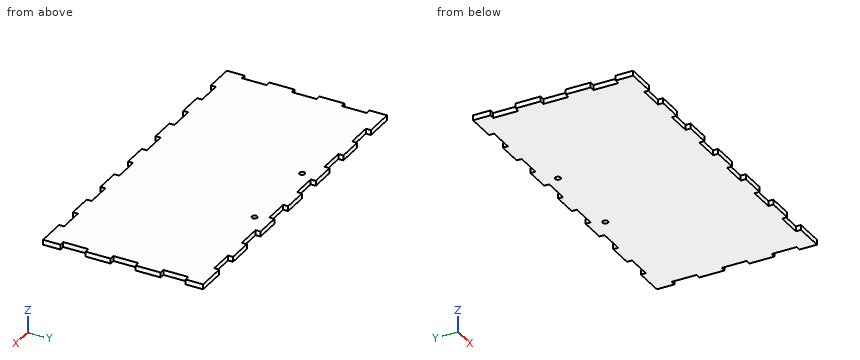
Autodesk Inventor part; units mm, degrees
ref_plane "Work Plane1" through (0, 0, 0) normal (0, 0, 1) x (1, 0, 0)
ref_plane "YZ Plane" through (0, 0, 0) normal (1, 0, 0) x (0, 1, 0)
ref_plane "XZ Plane" through (0, 0, 0) normal (0, 1, 0) x (-1, 0, 0)
ref_plane "Work Plane1" through (0, 0, 0) normal (0, 0, 1) x (1, 0, 0)
sketch "Sketch1" plane through (0, 0, 0) normal (0, 0, 1) x (1, 0, 0)
  line L0 (0, -5) -> (43, -5)
  line L1 (0, -25) -> (0, -5)
  line L2 (0, -25) -> (3, -25)
  line L3 (3, -25) -> (43, -25)
  line L4 (43, -5) -> (43, -25)
  line L5 (127, -5) -> (170, -5)
  line L6 (127, -5) -> (127, -25)
  line L7 (167, -25) -> (127, -25)
  line L8 (170, -25) -> (167, -25)
  line L9 (170, -25) -> (170, -5)
  ellipse E0 centre (272.0385, -161.4535) end of major axis (262.0385, -161.4535) minor radius 9.7437
  line L10 (264.0385, -174.9547) -> (285, -186.7467)
  line L11 (285, -186.7467) -> (285, -136.1602)
  line L12 (285, -136.1602) -> (264.0385, -147.9522)
  ellipse E1 centre (272.0385, -161.4535) end of major axis (256.0385, -161.4535) minor radius 15.5899 (264.0385, -147.9522) -> (264.0385, -174.9547) ccw
  ellipse E2 centre (-102.0385, -161.4535) end of major axis (-92.0385, -161.4535) minor radius 9.7437
  line L13 (-94.0385, -174.9547) -> (-115, -186.7467)
  ellipse E3 centre (-102.0385, -161.4535) end of major axis (-86.0385, -161.4535) minor radius 15.5899 (-94.0385, -174.9547) -> (-94.0385, -147.9522) ccw
  line L14 (-115, -136.1602) -> (-94.0385, -147.9522)
  line L15 (-115, -186.7467) -> (-115, -136.1602)
  line L16 (-115, -136.1602) -> (-115, -5) construction
  line L17 (-115, -5) -> (285, -5) construction
  line L18 (285, -5) -> (285, -186.7467) construction
  line L19 (285, -186.7467) -> (-115, -186.7467) construction
  line L20 (-115, -186.7467) -> (-115, -136.1602) construction
  line L21 (285, -5) -> (-115, -5)
  line L22 (-115, -5) -> (-115, -186.7467)
  line L23 (-115, -186.7467) -> (285, -186.7467)
  line L24 (285, -186.7467) -> (285, -5)
  circle A0 centre (147, -15) radius 3.25
  circle A1 centre (23, -15) radius 3.25
  circle A2 centre (23, -15) radius 2.4585
  circle A3 centre (147, -15) radius 2.4585
  line L25 (-115, -5) -> (285, -5)
  line L26 (285, -5) -> (285, 5)
  line L27 (285, 5) -> (-115, 5)
  line L28 (-115, 5) -> (-115, -5)
  point P0 (0, 0)
  point P1 (170, -15)
  point P2 (147, -25)
  point P3 (23, -25)
  point P4 (43, -15)
  dimension "d0" = 6.5
  dimension "d2" = 10
extrude "Plate1" add sketch "Sketch1" along normal blind 6 contours L21 L28 L27 L26 L5 L0 | L0 L4 L3 L2 L1 | L1 L2 L3 L4 L21 L6 L7 L8 L9 L24 L12 E1 L10 L23 L13 E3 L14 L22 | L5 L9 L8 L7 L6 | L14 E3 L13 L15 | L10 E1 L12 L11 | E0 | E2 | A0 | A1 | A2 | A3
sketch "Sketch2" plane through (0, 0, 6) normal (0, 0, 1) x (1, 0, 0)
  line L0 (-115, -186.7467) -> (-115, 5)
  line L1 (285, -186.7467) -> (-115, -186.7467)
  line L2 (285, 5) -> (285, -186.7467)
  line L3 (-115, 5) -> (285, 5)
  line L4 (285, -186.7467) -> (285, 5)
  line L5 (285, -75.8734) -> (279, -75.8734)
  line L6 (279, -75.8734) -> (279, -105.8734)
  line L7 (279, -105.8734) -> (285, -105.8734)
  line L8 (285, -105.8734) -> (285, -75.8734)
  line L9 (285, -45.8734) -> (279, -45.8734)
  line L10 (279, -45.8734) -> (279, -15.8734)
  line L11 (279, -15.8734) -> (285, -15.8734)
  line L12 (285, -15.8734) -> (285, -45.8734)
  line L13 (285, -135.8734) -> (279, -135.8734)
  line L14 (279, -135.8734) -> (279, -165.8734)
  line L15 (279, -165.8734) -> (285, -165.8734)
  line L16 (285, -165.8734) -> (285, -135.8734)
  line L17 (285, 5) -> (-115, 5) construction
  line L18 (85, 5) -> (85, -186.7467) construction
  line L19 (-115, -75.8734) -> (-109, -75.8734)
  line L20 (-109, -75.8734) -> (-109, -105.8734)
  line L21 (-109, -105.8734) -> (-115, -105.8734)
  line L22 (-115, -105.8734) -> (-115, -75.8734)
  line L23 (-115, -45.8734) -> (-109, -45.8734)
  line L24 (-109, -45.8734) -> (-109, -15.8734)
  line L25 (-109, -15.8734) -> (-115, -15.8734)
  line L26 (-115, -15.8734) -> (-115, -45.8734)
  line L27 (-115, -135.8734) -> (-109, -135.8734)
  line L28 (-109, -135.8734) -> (-109, -165.8734)
  line L29 (-109, -165.8734) -> (-115, -165.8734)
  line L30 (-115, -165.8734) -> (-115, -135.8734)
  line L31 (-115, -186.7467) -> (285, -186.7467)
  line L32 (250, -186.7467) -> (220, -186.7467)
  line L33 (220, -186.7467) -> (220, -180.7467)
  line L34 (220, -180.7467) -> (250, -180.7467)
  line L35 (250, -180.7467) -> (250, -186.7467)
  line L36 (190, -186.7467) -> (160, -186.7467)
  line L37 (160, -186.7467) -> (160, -180.7467)
  line L38 (160, -180.7467) -> (190, -180.7467)
  line L39 (190, -180.7467) -> (190, -186.7467)
  line L40 (130, -186.7467) -> (100, -186.7467)
  line L41 (100, -186.7467) -> (100, -180.7467)
  line L42 (100, -180.7467) -> (130, -180.7467)
  line L43 (130, -180.7467) -> (130, -186.7467)
  line L44 (285, -90.8734) -> (-115, -90.8734) construction
  line L45 (250, 5) -> (220, 5)
  line L46 (220, 5) -> (220, -1)
  line L47 (220, -1) -> (250, -1)
  line L48 (250, -1) -> (250, 5)
  line L49 (190, 5) -> (160, 5)
  line L50 (160, 5) -> (160, -1)
  line L51 (160, -1) -> (190, -1)
  line L52 (190, -1) -> (190, 5)
  line L53 (130, 5) -> (100, 5)
  line L54 (100, 5) -> (100, -1)
  line L55 (100, -1) -> (130, -1)
  line L56 (130, -1) -> (130, 5)
  circle A0 centre (23, -15) radius 3.25
  line L57 (-80, -186.7467) -> (-50, -186.7467)
  line L58 (-50, -186.7467) -> (-50, -180.7467)
  line L59 (-50, -180.7467) -> (-80, -180.7467)
  line L60 (-80, -180.7467) -> (-80, -186.7467)
  line L61 (-20, -186.7467) -> (10, -186.7467)
  line L62 (10, -186.7467) -> (10, -180.7467)
  line L63 (10, -180.7467) -> (-20, -180.7467)
  line L64 (-20, -180.7467) -> (-20, -186.7467)
  line L65 (40, -186.7467) -> (70, -186.7467)
  line L66 (70, -186.7467) -> (70, -180.7467)
  line L67 (70, -180.7467) -> (40, -180.7467)
  line L68 (40, -180.7467) -> (40, -186.7467)
  line L69 (70, 5) -> (70, -1)
  line L70 (40, 5) -> (70, 5)
  line L71 (40, -1) -> (40, 5)
  line L72 (10, 5) -> (10, -1)
  line L73 (-20, 5) -> (10, 5)
  line L74 (10, -1) -> (-20, -1)
  line L75 (-20, -1) -> (-20, 5)
  line L76 (70, -1) -> (40, -1)
  line L77 (-50, 5) -> (-50, -1)
  line L78 (-80, 5) -> (-50, 5)
  line L79 (-80, -1) -> (-80, 5)
  line L80 (-50, -1) -> (-80, -1)
  point P0 (0, 0)
  point P1 (115, -180.7467)
  point P2 (115, -1)
  point P3 (55, -180.7467)
  point P4 (55, -1)
  dimension "d3" = 6
  dimension "d4" = 30
  dimension "d5" = 30
  dimension "d6" = 30
  dimension "d7" = 30
  dimension "d8" = 30
  dimension "d10" = 15
extrude "Cut1" cut sketch "Sketch2" against normal blind 6 contours L0 L27 L28 L29 | L60 L59 L58 L1 | L0 L19 L20 L21 | L64 L63 L62 L1 | L0 L25 L24 L23 | L68 L67 L66 L1 | L41 L42 L43 L1 | L3 L77 L80 L79 | L37 L38 L39 L1 | L3 L72 L74 L75 | L33 L34 L35 L1 | L3 L69 L76 L71 | L3 L56 L55 L54 | L15 L14 L13 L2 | L3 L52 L51 L50 | L7 L6 L5 L2 | L3 L48 L47 L46 | L9 L10 L11 L2
sketch "Sketch3" plane through (0, 0, 0) normal (0, 0, -1) x (-1, 0, 0)
  circle A0 centre (-147, -15) radius 3.25
  circle A1 centre (-23, -15) radius 3.25
  circle A2 centre (-136.75, -15) radius 3.25
  circle A3 centre (-33.25, -15) radius 3.25
  line L0 (115, -5) -> (-285, -5) construction
  line L1 (-136.75, -15) -> (-33.25, -15) construction
  point P0 (0, 0)
  point P1 (-23, -15)
  point P2 (-85, -15)
  point P3 (-85, -5)
  dimension "d13" = 103.5
extrude "Cut2" cut sketch "Sketch3" against normal blind 6 contours A2 | A3
equation "\"d5\" = d4"
equation "\"d6\" = d5"
equation "\"d7\" = d4"
equation "\"d8\" = d7"
equation "\"d11\" = Thickness"
equation "\"d14\" = Thickness"
equation "\"d1\" = Thickness"
equation "\"BendRadius\" = Thickness"
equation "\"BendReliefWidth\" = Thickness"
equation "\"BendReliefDepth\" = 0.5 * Thickness"
equation "\"CornerReliefSize\" = 4 * Thickness"
equation "\"MinimumRemnant\" = 2 * Thickness"
equation "\"TransitionRadius\" = BendRadius"
equation "\"JacobiRadiusSize\" = BendRadius"
equation "\"GapSize\" = Thickness"
properties part number "elektronica behuizing" material "Wood (Birch)"
Design review of the part built by this model. Coordinates are the model's own, in mm. Coordinates: 2 decimals unless noted, no trailing zeros. Loops run counter-clockwise (first coordinate to the right, second up) from the corner with the lowest first, then second, coordinate; pieces in that order, holes last. Notation, with made-up numbers: (7.25, 47.25) -> (51.25, 47.25) arc R14 cw to (51.25, 59.25) -> close; hole circle Ø2 at (71, -11). An arc over 180 degrees is marked (long way). Use a Markdown table: item, result. Add a question column.
Item 1: We need section A-A, the plane z = 2. Count the separate pieces of the cut face and the enclosed holes in it, and give its area (3 significant figures).
Item 2: Clearance check with flat-ended pins moving along their axes: P1, Ø3, axis at x = 117.5, z = 2.5, coming from the -Y side; P2, Ø3, axis at y = -37.5, z = 1, coming from the -X side. State where each tip first meets the part, or that it passes through.
Item 3: We need section B-B, the plane x = 227.5. Write out the cut boundary in (y, z), and give its area (3 significant figures).
Item 4: Wall thickness on L1, parallel to Y at x = 33.25, z = 1.45; L2, parallel to X at y = -93.5, z = 3.5; L3, parallel to Y at x = -54.5, z = 1.9: over which ranges is each line inside the solid? List them lowest first. Write a range as from..to.
Numbers:
| question | item | result |
|---|---|---|
| 1 | separate pieces | 1 |
| 1 | enclosed holes | 2 |
| 1 | area | 73,400 mm^2 |
| 2 | P1 | stops at y = -180.75 |
| 2 | P2 | stops at x = -109 |
| 3 | outline | (-180.75, 0) -> (-1, 0) -> (-1, 6) -> (-180.75, 6) -> close |
| 3 | area | 1,080 mm^2 |
| 4 | L1 | y = -186.75..-18.25, -11.75..5 |
| 4 | L2 | x = -109..279 |
| 4 | L3 | y = -180.75..-1 |
